```python
from build123d import *
from OCP.BRepFilletAPI import BRepFilletAPI_MakeChamfer

# Parameters (mm, degrees)
SKETCH1_R           = 3.85
BOSS_EXTRUDE1_DEPTH = 4.5
SKETCH2_W           = 9
SKETCH2_H           = 10.5
BOSS_EXTRUDE2_DEPTH = 13
CHAMFER1_SIZE       = 0.9
CHAMFER1_SIZE2      = 1.558845727
SKETCH3_W           = 1.6
SKETCH3_H           = 0.3
SKETCH3_W_2         = 0.3
SKETCH3_H_2         = 1.6
BOSS_EXTRUDE3_DEPTH = 5
CHAMFER2_SIZE       = 0.6
CHAMFER2_SIZE2      = 0.346410162
SKETCH4_R           = 1.85
CUT_EXTRUDE1_DEPTH  = 17.5
CHAMFER3_SIZE       = 0.5


with BuildPart() as part:
    # Sketch1 → Boss-Extrude1 (new body)
    with BuildSketch(Plane.XY):
        Circle(SKETCH1_R)
    extrude(amount=BOSS_EXTRUDE1_DEPTH)

    # Sketch2 → Boss-Extrude2 (add)
    with BuildSketch(Plane(origin=(0, 0, 0), x_dir=(-1, 0, 0), z_dir=(0, 0, -1))):
        with Locations((0, -0.3)):
            Rectangle(SKETCH2_W, SKETCH2_H)
    extrude(amount=BOSS_EXTRUDE2_DEPTH)

    # Chamfer1: one chamfer whose edges measure the first distance from different faces: ONE call of the kernel's chamfer builder (chamfer() names one face for all edges)
    chamfer1_edges_1 = [part.edges().sort_by_distance(p)[0] for p in [
        (-4.5, 4.95, -6.5),
    ]]
    chamfer1_side_1 = [part.faces().sort_by_distance(p)[0] for p in [
        (-4.5, -0.3, -6.5),
    ]]
    chamfer1_edges_2 = [part.edges().sort_by_distance(p)[0] for p in [
        (4.5, 4.95, -6.5),
    ]]
    chamfer1_side_2 = [part.faces().sort_by_distance(p)[0] for p in [
        (4.5, -0.3, -6.5),
    ]]
    chamfer1 = BRepFilletAPI_MakeChamfer(part.part.solid().wrapped)
    for e in chamfer1_edges_1:
        chamfer1.Add(CHAMFER1_SIZE, CHAMFER1_SIZE2, e.wrapped, chamfer1_side_1[0].wrapped)  # the first distance lies on this face
    for e in chamfer1_edges_2:
        chamfer1.Add(CHAMFER1_SIZE, CHAMFER1_SIZE2, e.wrapped, chamfer1_side_2[0].wrapped)  # the first distance lies on this face
    add(Compound.cast(chamfer1.Shape()), mode=Mode.REPLACE)

    # Sketch3 → Boss-Extrude3 (add)
    with BuildSketch(Plane(origin=(0, 0, -13), x_dir=(-1, 0, 0), z_dir=(0, 0, -1))):
        with Locations((0, 4)):
            Rectangle(SKETCH3_W, SKETCH3_H)
        with Locations((3.55, 0)):
            Rectangle(SKETCH3_W_2, SKETCH3_H_2)
        with Locations((-3.55, 0)):
            Rectangle(SKETCH3_W_2, SKETCH3_H_2)
        with Locations((0, -4.6)):
            Rectangle(SKETCH3_W, SKETCH3_H)
    extrude(amount=BOSS_EXTRUDE3_DEPTH)

    # Chamfer2: one chamfer whose edges measure the first distance from different faces: ONE call of the kernel's chamfer builder (chamfer() names one face for all edges)
    chamfer2_edges_1 = [part.edges().sort_by_distance(p)[0] for p in [
        (0.8, 4, -18),
    ]]
    chamfer2_side_1 = [part.faces().sort_by_distance(p)[0] for p in [
        (0.8, 4, -15.5),
    ]]
    chamfer2_edges_2 = [part.edges().sort_by_distance(p)[0] for p in [
        (-0.8, 4, -18),
    ]]
    chamfer2_side_2 = [part.faces().sort_by_distance(p)[0] for p in [
        (-0.8, 4, -15.5),
    ]]
    chamfer2_edges_3 = [part.edges().sort_by_distance(p)[0] for p in [
        (-3.55, -0.8, -18),
    ]]
    chamfer2_side_3 = [part.faces().sort_by_distance(p)[0] for p in [
        (-3.55, -0.8, -15.5),
    ]]
    chamfer2_edges_4 = [part.edges().sort_by_distance(p)[0] for p in [
        (-3.55, 0.8, -18),
    ]]
    chamfer2_side_4 = [part.faces().sort_by_distance(p)[0] for p in [
        (-3.55, 0.8, -15.5),
    ]]
    chamfer2_edges_5 = [part.edges().sort_by_distance(p)[0] for p in [
        (3.55, -0.8, -18),
    ]]
    chamfer2_side_5 = [part.faces().sort_by_distance(p)[0] for p in [
        (3.55, -0.8, -15.5),
    ]]
    chamfer2_edges_6 = [part.edges().sort_by_distance(p)[0] for p in [
        (3.55, 0.8, -18),
    ]]
    chamfer2_side_6 = [part.faces().sort_by_distance(p)[0] for p in [
        (3.55, 0.8, -15.5),
    ]]
    chamfer2_edges_7 = [part.edges().sort_by_distance(p)[0] for p in [
        (0.8, -4.6, -18),
    ]]
    chamfer2_side_7 = [part.faces().sort_by_distance(p)[0] for p in [
        (0.8, -4.6, -15.5),
    ]]
    chamfer2_edges_8 = [part.edges().sort_by_distance(p)[0] for p in [
        (-0.8, -4.6, -18),
    ]]
    chamfer2_side_8 = [part.faces().sort_by_distance(p)[0] for p in [
        (-0.8, -4.6, -15.5),
    ]]
    chamfer2 = BRepFilletAPI_MakeChamfer(part.part.solid().wrapped)
    for e in chamfer2_edges_1:
        chamfer2.Add(CHAMFER2_SIZE, CHAMFER2_SIZE2, e.wrapped, chamfer2_side_1[0].wrapped)  # the first distance lies on this face
    for e in chamfer2_edges_2:
        chamfer2.Add(CHAMFER2_SIZE, CHAMFER2_SIZE2, e.wrapped, chamfer2_side_2[0].wrapped)  # the first distance lies on this face
    for e in chamfer2_edges_3:
        chamfer2.Add(CHAMFER2_SIZE, CHAMFER2_SIZE2, e.wrapped, chamfer2_side_3[0].wrapped)  # the first distance lies on this face
    for e in chamfer2_edges_4:
        chamfer2.Add(CHAMFER2_SIZE, CHAMFER2_SIZE2, e.wrapped, chamfer2_side_4[0].wrapped)  # the first distance lies on this face
    for e in chamfer2_edges_5:
        chamfer2.Add(CHAMFER2_SIZE, CHAMFER2_SIZE2, e.wrapped, chamfer2_side_5[0].wrapped)  # the first distance lies on this face
    for e in chamfer2_edges_6:
        chamfer2.Add(CHAMFER2_SIZE, CHAMFER2_SIZE2, e.wrapped, chamfer2_side_6[0].wrapped)  # the first distance lies on this face
    for e in chamfer2_edges_7:
        chamfer2.Add(CHAMFER2_SIZE, CHAMFER2_SIZE2, e.wrapped, chamfer2_side_7[0].wrapped)  # the first distance lies on this face
    for e in chamfer2_edges_8:
        chamfer2.Add(CHAMFER2_SIZE, CHAMFER2_SIZE2, e.wrapped, chamfer2_side_8[0].wrapped)  # the first distance lies on this face
    add(Compound.cast(chamfer2.Shape()), mode=Mode.REPLACE)

    # Sketch4 → Cut-Extrude1 (cut)
    with BuildSketch(Plane.XY.offset(4.5)):
        Circle(SKETCH4_R)
    extrude(amount=-CUT_EXTRUDE1_DEPTH, mode=Mode.SUBTRACT)

    # Chamfer3
    chamfer3_edges = [part.edges().sort_by_distance(p)[0] for p in [
        (-1.85, 0, 4.5),
    ]]
    chamfer(chamfer3_edges, length=CHAMFER3_SIZE)


solid = part.part
```
Geometry check sheet. Reference: the model listing, model coordinates, mm. A direction names the side the tool comes from. Coordinates: 2 decimals unless noted, no trailing zeros. Loops run counter-clockwise (first coordinate to the right, second up) from the corner with the lowest first, then second, coordinate; pieces in that order, holes last. Notation, with made-up numbers: (41.5, 59.25) - (71.5, 59.25) arc R20 ccw to (71.5, 89.25) - close; hole circle Ø8 at (-34.75, 4.5). An arc over 180 degrees is marked (long way). One line per item, written item: value. Start each with the question number.
(1) Material ranges on line 1 (Y direction, x = 0, z = -2.75); line 2 (X direction, y = 0.5, z = -14.5); line 3 (X direction, y = -1.5, z = -8.25), recorded low to high. Write a range as [from, to].
(2) Mould release check, pull along X, two halves, no side actions. Record for faces 1 (the cylindrical face through (-0.401, -1.806, -4.381)), 2 (the flat face through (0, -5.55, -6)), 3 (the flat face through (-4.5, -1, -6)), 4 (the flat face through (-3.4, 0, -15)): released by +X, released by -X, zero draft, split by the parting line, or undercut.
(3) Tool access check on faces 5 (the flat face through (0, -4.45, -15)), 6 (the flat face through (0, 4.15, -15)), 7 (the cylindrical face through (-0.83, -3.76, 2.22)). Record the directions out of +Z, -Z, +X, -X, +Y, -Y that give a thin tool (end or side, any length) a straight path to the whole face; none if there is none.
(4) Cross-section at B-B on z = -13.25. Enter the section's corners in (x, y), plus the area to 3 significant figures.
(5) Depth check by flat-ended pin: P1, Ø1.8, axis at x = 0, z = -16, coming from the -Y side; P2, Ø2, axis at x = 1, y = -3, coming from the -Z side; P3, Ø0.5, axis at y = 0, z = -16.5, coming from the -X side. Enter the tip coordinate at first touch or a pass-through.
(6) Cross-section at D-D on z = -9.25. Enter the section's corners in (x, y).
(7) Cross-section at C-C on x = 0. Enter the section's corners in (y, z).
(8) Cross-section at A-A on y = 0. Enter the section's corners in (x, z), plus the area to 4 significant figures.
Results below:
1. line 1: y = [-5.55, -1.85], [1.85, 4.95]
1. line 2: x = [-3.7, -3.4], [3.4, 3.7]
1. line 3: x = [-4.5, -1.08], [1.08, 4.5]
2. face 1: undercut
2. face 2: zero draft
2. face 3: released by -X
2. face 4: undercut
3. face 5: -Z, +X, -X
3. face 6: -Z, +X, -X, +Y
3. face 7: +Z
4. outline: (-3.7, -0.8) - (-3.4, -0.8) - (-3.4, 0.8) - (-3.7, 0.8) - close; (-0.8, -4.75) - (0.8, -4.75) - (0.8, -4.45) - (-0.8, -4.45) - close; (-0.8, 3.85) - (0.8, 3.85) - (0.8, 4.15) - (-0.8, 4.15) - close; (3.4, -0.8) - (3.7, -0.8) - (3.7, 0.8) - (3.4, 0.8) - close
4. area: 1.92 mm2
5. P1: stops at y = -4.75
5. P2: stops at z = -13
5. P3: stops at x = -3.7
6. outline: (-4.5, -5.55) - (4.5, -5.55) - (4.5, 4.05) - (2.94, 4.95) - (-2.94, 4.95) - (-4.5, 4.05) - close; hole circle Ø3.7 at (0, 0)
7. outline: (-5.55, -13) - (-4.75, -13) - (-4.75, -18) - (-4.45, -18) - (-4.45, -13) - (-1.85, -13) - (-1.85, 4) - (-2.35, 4.5) - (-3.85, 4.5) - (-3.85, 0) - (-5.55, 0) - close; (1.85, -13) - (3.85, -13) - (3.85, -18) - (4.15, -18) - (4.15, -13) - (4.95, -13) - (4.95, 0) - (3.85, 0) - (3.85, 4.5) - (2.35, 4.5) - (1.85, 4) - close
8. outline: (-4.5, -13) - (-3.7, -13) - (-3.7, -18) - (-3.4, -18) - (-3.4, -13) - (-1.85, -13) - (-1.85, 4) - (-2.35, 4.5) - (-3.85, 4.5) - (-3.85, 0) - (-4.5, 0) - close; (1.85, -13) - (3.4, -13) - (3.4, -18) - (3.7, -18) - (3.7, -13) - (4.5, -13) - (4.5, 0) - (3.85, 0) - (3.85, 4.5) - (2.35, 4.5) - (1.85, 4) - close
8. area: 89.65 mm2
